CAD build for the part. Positions are in the model's coordinates, mm. Round coordinates to 2 decimals unless told otherwise and drop trailing zeros. Order: outer loops, then holes, each group sorted by start corner. A loop starts at its lowest first (then second) coordinate and runs counter-clockwise, first axis right, second up. Notation, with made-up numbers: (-22.75, 11.25) -> (-3.75, 11.25) arc R20 ccw to (-3.75, 47.25) -> close; hole circle Ø2 at (55, -4.75). An arc over 180 degrees is marked (long way). Return JSON: item names as keys, results as strings. Group by question number.
Q1. Probe line 1 along Y through (x, z) = (5.25, 79.5); line 2 along X through (y, z) = (5.5, 23); line 3 along X through (y, z) = (-1.5, 40). List the from-to ranges inside material, lowest first.
Q2. Cut at B-B (y = -1.75). Write the cut outline in (x, z).
Q3. Cut at A-A (z = -15.5). Write the cut outline in (x, y), then the cut area to 3 significant figures.
Q4. Flat gauge pins, fed straight in: pin 1 (5 mm diameter, centred on y = 5, z = -33.5, fed in from +X); pin 2 (1.5 mm diameter, centred on y = -3.5, z = -26.5, fed in from +X); pin 3 (1 mm diameter, centred on y = -4.5, z = -56.5, fed in from -X). Where does each tip first touch, or does it go through?
from build123d import *

# Parameters (mm, degrees)
BOSS_EXTRUDE1_DEPTH = 88.9


with BuildPart() as part:
    # Sketch1 → Boss-Extrude1 (new, symmetric)
    with BuildSketch(Plane.XY):
        with BuildLine():
            Line((-7.171036753, -0.254), (-3.805488829, -6.0833))
            ThreePointArc((-3.805488829, -6.0833), (-3.619547924, -6.269240905), (-3.365547924, -6.3373))
            Line((-3.365547924, -6.3373), (3.365547924, -6.3373))
            ThreePointArc((3.365547924, -6.3373), (3.619547924, -6.269240905), (3.805488829, -6.0833))
            Line((3.805488829, -6.0833), (7.171036753, -0.254))
            ThreePointArc((7.171036753, -0.254), (7.239095848, 0), (7.171036753, 0.254))
            Line((7.171036753, 0.254), (3.805488829, 6.0833))
            ThreePointArc((3.805488829, 6.0833), (3.619547924, 6.269240905), (3.365547924, 6.3373))
            Line((3.365547924, 6.3373), (-3.365547924, 6.3373))
            ThreePointArc((-3.365547924, 6.3373), (-3.619547924, 6.269240905), (-3.805488829, 6.0833))
            Line((-3.805488829, 6.0833), (-7.171036753, 0.254))
            ThreePointArc((-7.171036753, 0.254), (-7.239095848, 0), (-7.171036753, -0.254))
        make_face()
    extrude(amount=BOSS_EXTRUDE1_DEPTH, both=True)


solid = part.part
Solution:
{
 "1": {"line 1": "y = -3.58 to 3.58", "line 2": "x = -4.14 to 4.14", "line 3": "x = -6.45 to 6.45"},
 "2": {"outline": "(-6.31, -88.9) -> (6.31, -88.9) -> (6.31, 88.9) -> (-6.31, 88.9) -> close"},
 "3": {"outline": "(-7.17, -0.25) -> (-3.81, -6.08) arc R0.51 ccw to (-3.37, -6.34) -> (3.37, -6.34) arc R0.51 ccw to (3.81, -6.08) -> (7.17, -0.25) arc R0.51 ccw to (7.17, 0.25) -> (3.81, 6.08) arc R0.51 ccw to (3.37, 6.34) -> (-3.37, 6.34) arc R0.51 ccw to (-3.81, 6.08) -> (-7.17, 0.25) arc R0.51 ccw to start", "area": "139 mm²"},
 "4": {"pin 1": "stops at x = 5.87", "pin 2": "stops at x = 5.73", "pin 3": "stops at x = -5.01"}
}
